Here's how the part is built. I have some questions about the finished solid (model axes, mm). A direction names the side the tool comes from. Coordinates: 2 decimals unless noted, no trailing zeros. Write each loop counter-clockwise with the first axis right and the second up, starting at its lowest first coordinate (ties: lowest second). Pieces come first, ordered by that corner, then holes. Notation, with made-up numbers: (-0.5, 7.5) -> (39.5, 7.5) arc R32 cw to (39.5, 43.5) -> close; hole circle Ø5 at (85.5, 76). An arc over 180 degrees is marked (long way). Put each result on its own line as item: value.
Autodesk Inventor part; units mm, degrees
ref_plane "YZ Plane" through (0, 0, 0) normal (1, 0, 0) x (0, 1, 0)
ref_plane "XZ Plane" through (0, 0, 0) normal (0, 1, 0) x (-1, 0, 0)
ref_plane "XY Plane" through (0, 0, 0) normal (0, 0, 1) x (1, 0, 0)
sketch "Boceto1" plane through (0, 0, 0) normal (0, 1, 0) x (-1, 0, 0)
  line L0 (7.2949, 12.862) -> (7.2949, -12.138)
  line L1 (7.2949, -12.138) -> (-32.7051, -12.138)
  line L2 (-32.7051, -12.138) -> (-32.7051, 12.862)
  line L3 (-32.7051, 12.862) -> (7.2949, 12.862)
  line L4 (-2.7051, -12.138) -> (-2.7051, 12.862)
  circle A0 centre (-17.7051, -7.138) radius 2
  circle A1 centre (-17.7051, 7.862) radius 2
  line L5 (7.2949, -12.138) -> (2.2949, -12.138)
  circle A2 centre (2.2949, -7.138) radius 2
  point P0 (0, 0)
  dimension "d0" = 25
  dimension "d1" = 40
  dimension "d11" = 4
  dimension "d12" = 4
  dimension "d13" = 5
  dimension "d14" = 5
  dimension "d15" = 15
  dimension "d16" = 15
  dimension "d18" = 4
  dimension "d19" = 5
  dimension "d20" = 5
extrude "Extrusión2" add sketch "Boceto1" along normal blind 2 contours L4 L1 L2 L3
extrude "Extrusión3" add sketch "Boceto1" along normal blind 2 contours L0 L1 L4 L3
bend part "Pieza de plegado1" radius 0.5 angle 90 line through (2.7051, 0, -12.138) along (0, 0, 1) centre toward (0, -1, 0) moving side (-1, 0, 0) both sides no
properties part number "leche"
Item 1: Imagine slicing it at C-C on x = 18. Write out the boundary of the cut face in (y, z).
Output:
outline: (0, -12.14) -> (2, -12.14) -> (2, -9.12) -> (0, -9.12) -> close; (0, -5.16) -> (2, -5.16) -> (2, 5.88) -> (0, 5.88) -> close; (0, 9.84) -> (2, 9.84) -> (2, 12.86) -> (0, 12.86) -> close
Item 2: Imagine slicing it at D-D on y = -2. Write out the boundary of the cut face in (x, z).
Output:
outline: (0.21, -12.14) -> (2.21, -12.14) -> (2.21, 12.86) -> (0.21, 12.86) -> close
Item 3: If we mould it in two halves opening along Z, with no side actions, what happens to faces 1 (the flat face through (12.9, 0.5, 12.862)), 2 (the cylindrical face through (15.797, 0.986, -7.739)), 3 (the flat face through (2.205, -5, 1)), 4 (the cylindrical face through (15.797, 0.986, 7.261))? For each: released by +Z, released by -Z, zero draft, split by the parting line, or undercut.
Output:
face 1: released by +Z
face 2: undercut
face 3: zero draft
face 4: undercut
Item 4: Which directions (+Z, -Z, +X, -X, +Y, -Y) give clear straight access to the entire face, cutting with the end or side of a thin tool? Please do faces 5 (the flat face through (32.705, 1, 0)), 6 (the flat face through (18, 0, 1)).
Output:
face 5: +Z, -Z, +X, +Y, -Y
face 6: +Z, -Z, +X, -Y
Item 5: Imagine slicing it at B-B on y = -3.5. Write out the boundary of the cut face in (x, z).
Output:
outline: (0.21, -12.14) -> (2.21, -12.14) -> (2.21, -8.73) -> (0.21, -8.73) -> close; (0.21, -5.55) -> (2.21, -5.55) -> (2.21, 12.86) -> (0.21, 12.86) -> close
Item 6: Please list where these lines run through material, in increasing order: line 1 along Y through (x, z) = (6, 1.5); line 2 along X through (y, z) = (-2.25, 4.5); line 3 along Y through (x, z) = (2, 9.75). Write a range as from..to.
Output:
line 1: y = 0..2
line 2: x = 0.21..2.21
line 3: y = -9.71..1.9
Item 7: Imagine slicing it at A-A on z = 7. Write out the boundary of the cut face in (x, y).
Output:
outline: (0.21, -9.71) -> (2.21, -9.71) -> (2.21, -0.5) arc R0.5 cw to (2.71, 0) -> (15.9, 0) -> (15.9, 2) -> (2.71, 2) arc R2.5 ccw to (0.21, -0.5) -> close; (19.51, 0) -> (32.71, 0) -> (32.71, 2) -> (19.51, 2) -> close
Item 8: For P1, Ø3, axis at x = 17.71, z = 7.86, coming from the +Y side (3 decimals); P2, Ø4.5, axis at y = -4.71, z = -7.14, coming from the +X side; P3, Ø2, axis at x = 12.5, z = 8.5, coming from the -Y side, each with a flat end and sliding along its axis, tell me the tip position at first contact or that it passes through.
Output:
P1: passes through
P2: stops at x = 2.21
P3: stops at y = 0
